Check sheet for the drawn part. Datum: minimum x, y, z corner. Units: mm. A direction names the side the tool comes from. Round coordinates to 2 decimals unless told otherwise and drop trailing zeros. Order: outer loops, then holes, each group sorted by start corner. A loop starts at its lowest first (then second) coordinate and runs counter-clockwise, first axis right, second up. Notation, with made-up numbers: M -28,12.5 L -1,12.5 A16 cw -1,43.5 Z; hole C 53,38.25 d5. An arc over 180 degrees is marked long. Use one line per item in the form item = value. Start each with the question number.
Item 1: Cross-section at A-A on z = 16.5. Enter the section's corners in (x, y).
Item 2: Cross-section at D-D on y = 2.25. Enter the section's corners in (x, z).
Item 3: Cross-section at C-C on x = 6.5. Enter the section's corners in (y, z), then the cut area to 3 significant figures.
Item 4: Go/stop test with flat-tipped pins: pin 1 Ø7 at (y, z) = (6, 15) entering from -X; pin 2 Ø1.5 at (x, y) = (3.5, 5.5) entering from +Z; pin 3 Ø2 at (x, y) = (7, 8) entering from -Z; pin 4 Ø4 at (x, z) = (3.5, 18) entering from -Y. Record where each tip stops, or that it passes through.
Item 5: Thickness scan on probe 1 along Z at (x, y) = (6.7, 7.5); probe 2 along Y at (x, z) = (7.3, 16.5); probe 3 along Z at (x, y) = (5.5, 13). Record the ranges inside material, lowest first. Write a range as [from, to].
Item 6: Cross-section at B-B on y = 7.5. Enter the section's corners in (x, z).
Item 7: Tool access check on the marked faces 1, 2 and 3. Record the directions out of +Z, -Z, +X, -X, +Y, -Y that give a thin tool (end or side, any length) a straight path to the whole face; none if there is none.
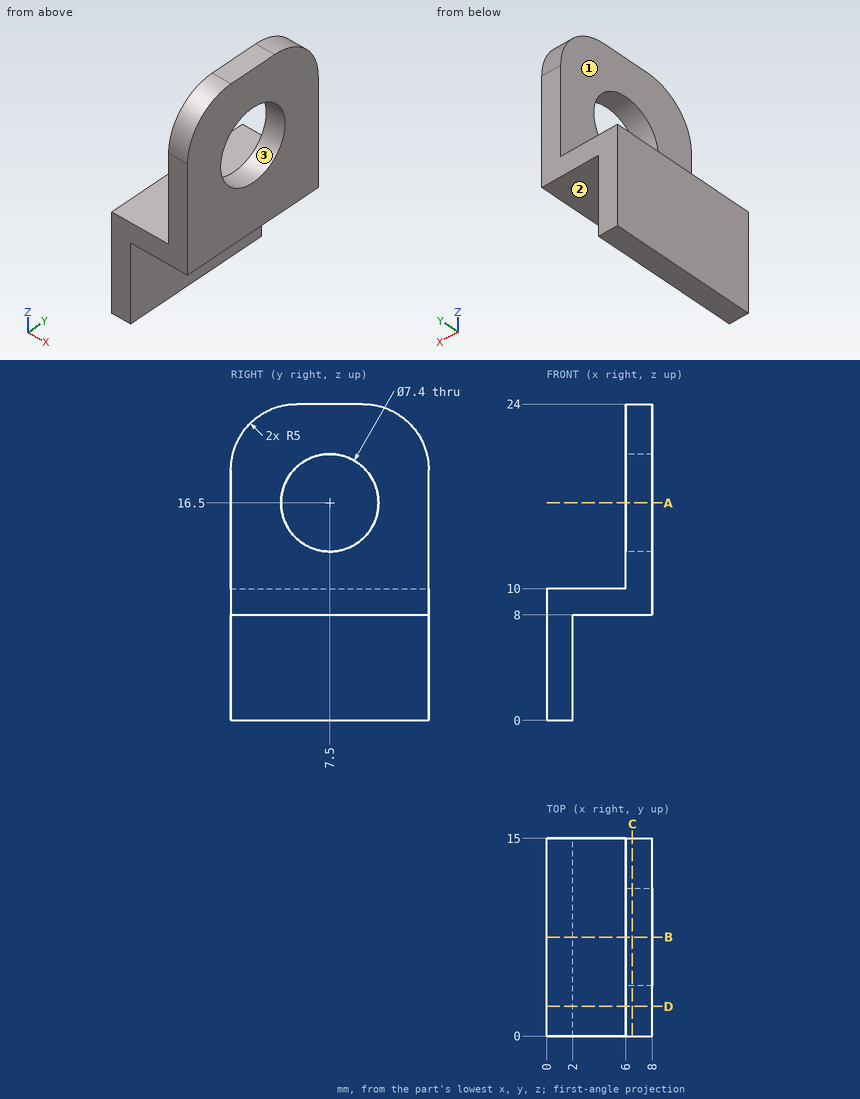
Output values:
q1.outline = M 6,0 L 8,0 L 8,3.8 L 6,3.8 Z; M 6,11.2 L 8,11.2 L 8,15 L 6,15 Z
q2.outline = M 0,0 L 2,0 L 2,8 L 8,8 L 8,23.18 L 6,23.18 L 6,10 L 0,10 Z
q3.outline = M 0,8 L 15,8 L 15,19 A5 ccw 10,24 L 5,24 A5 ccw 0,19 Z; hole C 7.5,16.5 d7.4
q3.area = 186 mm2
q4.pin_1 = 6
q4.pin_2 = 10
q4.pin_3 = 8
q4.pin_4 = through
q5.probe_1 = [8, 12.8], [20.2, 24]
q5.probe_2 = [0, 3.8], [11.2, 15]
q5.probe_3 = [8, 10]
q6.outline = M 0,0 L 2,0 L 2,8 L 8,8 L 8,12.8 L 6,12.8 L 6,10 L 0,10 Z; M 6,20.2 L 8,20.2 L 8,24 L 6,24 Z
q7.face_1 = +Z, -X, +Y, -Y
q7.face_2 = -Z, +X, +Y, -Y
q7.face_3 = +X, -X
